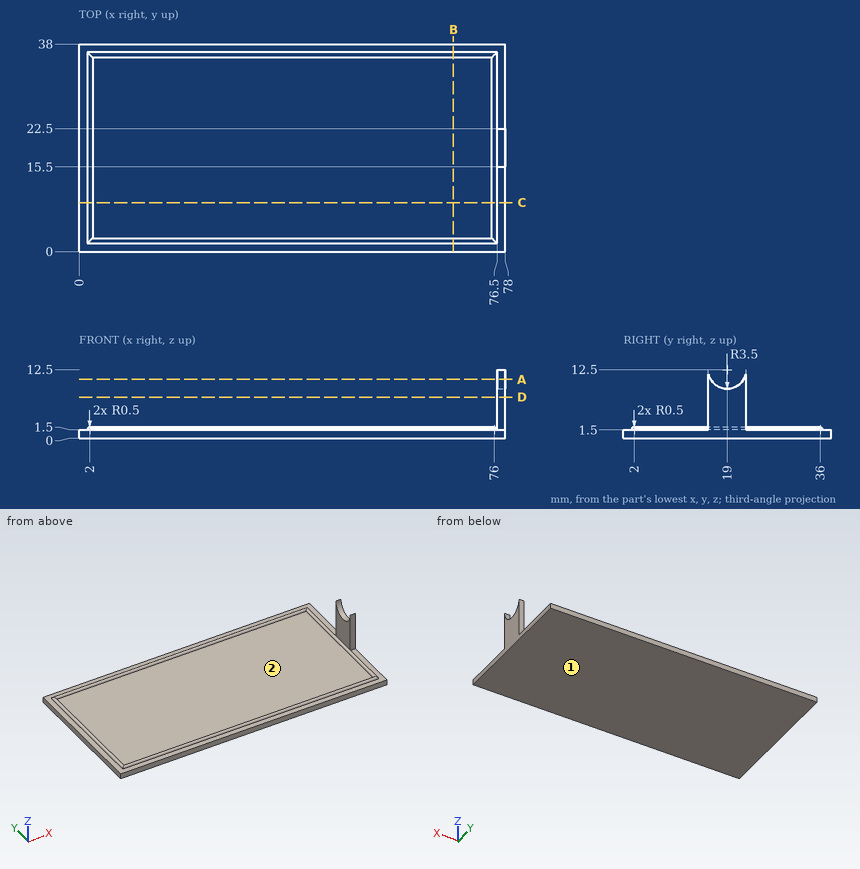
Part print with two shaded views. Sizes in mm from the minimum x, y, z corner. Give positions to 0.01 mm unless a question says otherwise; leave off trailing zeros. Order: outer loops, then holes, each group sorted by start corner. A loop starts at its lowest first (then second) coordinate and runs counter-clockwise, first axis right, second up. Notation, with made-up numbers: M -36,46.25 L 5,46.25 A27 cw 5,63.25 Z; hole C -0.75,8.25 d8. An arc over 180 degrees is marked long. Write item = value, one per line.
Q1. Flat gauge pins, fed straight in: pin 1 (1.5 mm diameter, centred on x = 43.5, z = 2.5, fed in from -Y); pin 2 (3.5 mm diameter, centred on y = 18.5, z = 7.5, fed in from -X); pin 3 (1.5 mm diameter, centred on x = 68, y = 21, fed in from -Z). Where does each tip first touch, or does it go through?
Derived:
pin_1 = 1.57
pin_2 = 76.5
pin_3 = 0
Q2. Drill centre lines: line 1 (Z direction, x = 64, y = 20); line 2 (Y direction, x = 24.5, z = 1.75); line 3 (X direction, y = 16.5, z = 3.75). Where is each one in solid material? Low to high. Write a range as [from, to].
Derived:
line_1 = [0, 1.5]
line_2 = [1.57, 2.43], [35.57, 36.43]
line_3 = [76.5, 78]
Q3. Cut at D-D, the plane z = 7.5. List the corners of the cut face in (x, y).
Derived:
outline = M 76.5,15.5 L 78,15.5 L 78,22.5 L 76.5,22.5 Z
Q4. Cut at A-A, the plane z = 10.75. List the corners of the cut face in (x, y).
Derived:
outline = M 76.5,15.5 L 78,15.5 L 78,15.97 L 76.5,15.97 Z; M 76.5,22.03 L 78,22.03 L 78,22.5 L 76.5,22.5 Z
Q5. Cut at C-C, the plane y = 9. List the corners of the cut face in (x, z), then the cut area to 3 significant figures.
Derived:
outline = M 0,0 L 78,0 L 78,1.5 L 76.5,1.5 A0.5 ccw 75.5,1.5 L 2.5,1.5 A0.5 ccw 1.5,1.5 L 0,1.5 Z
area = 118 mm2
Q6. Cut at B-B, the plane x = 68.5. List the corners of the cut face in (y, z), then the cut area to 3 significant figures.
Derived:
outline = M 0,0 L 38,0 L 38,1.5 L 36.5,1.5 A0.5 ccw 35.5,1.5 L 2.5,1.5 A0.5 ccw 1.5,1.5 L 0,1.5 Z
area = 57.8 mm2
Q7. Two-plate mould, pull along X, no slides. Class the marked faces 1 and 2: pulls with the +X half, pulls with the -X half, needs draft (parallel to the pull), parting line crosses it, or undercut.
Derived:
face_1 = needs draft
face_2 = undercut
